```python
from build123d import *

# Parameters (mm, degrees)
SKETCH_1_R        = 1
EXTRUDE_1_DEPTH   = 3
SKETCH_2_R        = 4.35
SKETCH_2_R_2      = 3.35
EXTRUDE_1_2_DEPTH = 3


with BuildPart() as part:
    # 草图1 → Extrude 1 (new body)
    with BuildSketch(Plane.XY):
        with BuildLine():
            Line((-2.470698832, 13.581637634), (-3.604292918, 6.242818459))
            Line((-3.604292918, 6.242818459), (-10.5266938, 8.93050677))
            ThreePointArc((-10.5266938, 8.93050677), (-13.596598839, 7.85), (-12.997392632, 4.651130864))
            Line((-12.997392632, 4.651130864), (-7.208585836, 0))
            Line((-7.208585836, 0), (-12.997392632, -4.651130864))
            ThreePointArc((-12.997392632, -4.651130864), (-13.596598839, -7.85), (-10.5266938, -8.93050677))
            Line((-10.5266938, -8.93050677), (-3.604292918, -6.242818459))
            Line((-3.604292918, -6.242818459), (-2.470698832, -13.581637634))
            ThreePointArc((-2.470698832, -13.581637634), (0, -15.7), (2.470698832, -13.581637634))
            Line((2.470698832, -13.581637634), (3.604292918, -6.242818459))
            Line((3.604292918, -6.242818459), (10.5266938, -8.93050677))
            ThreePointArc((10.5266938, -8.93050677), (13.596598839, -7.85), (12.997392632, -4.651130864))
            Line((12.997392632, -4.651130864), (7.208585836, 0))
            Line((7.208585836, 0), (12.997392632, 4.651130864))
            ThreePointArc((12.997392632, 4.651130864), (13.596598839, 7.85), (10.5266938, 8.93050677))
            Line((10.5266938, 8.93050677), (3.604292918, 6.242818459))
            Line((3.604292918, 6.242818459), (2.470698832, 13.581637634))
            ThreePointArc((2.470698832, 13.581637634), (0, 15.7), (-2.470698832, 13.581637634))
        make_face()
        with Locations((6.495190528, 3.75)):
            Circle(SKETCH_1_R, mode=Mode.SUBTRACT)
        with Locations((0, 7.5)):
            Circle(SKETCH_1_R, mode=Mode.SUBTRACT)
        with Locations((6.495190528, -3.75)):
            Circle(SKETCH_1_R, mode=Mode.SUBTRACT)
        with Locations((0, -7.5)):
            Circle(SKETCH_1_R, mode=Mode.SUBTRACT)
        with Locations((-6.495190528, -3.75)):
            Circle(SKETCH_1_R, mode=Mode.SUBTRACT)
        with Locations((-6.495190528, 3.75)):
            Circle(SKETCH_1_R, mode=Mode.SUBTRACT)
    extrude(amount=EXTRUDE_1_DEPTH)

    # 草图2 → Extrude 1 2 (add)
    with BuildSketch(Plane.XY.offset(3)):
        Circle(SKETCH_2_R)
        Circle(SKETCH_2_R_2, mode=Mode.SUBTRACT)
    extrude(amount=EXTRUDE_1_2_DEPTH)


solid = part.part
```
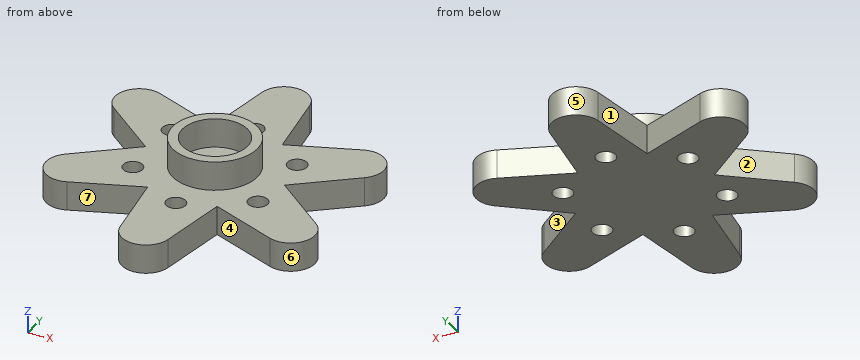
Geometry check sheet. Reference: the model listing, model coordinates, mm. Face numbers are marked on the shaded views. A direction names the side the tool comes from. Coordinates: 2 decimals unless noted, no trailing zeros. Order: outer loops, then holes, each group sorted by start corner. A loop starts at its lowest first (then second) coordinate and runs counter-clockwise, first axis right, second up. Notation, with made-up numbers: (1.5, -13) - (25.5, -13) arc R28 ccw to (25.5, 12) - close; hole circle Ø10 at (-8, 47.5). An arc over 180 degrees is marked (long way). Answer in a Markdown table with one row per item. Add a question column.
1. Section check A-A (z = 0.7). Enter the section's corners in (x, y), plus the area to 3 significant figures.
2. Gauge pin test, flat ends, axial feed: pin 1 Ø6 at (x, y) = (7.5, -5) entering from +Z; pin 2 Ø1.6 at (x, y) = (0, 7.5) entering from -Z. Record the tip position at first contact, or that the pin passes through.
3. Section check B-B (x = 0). Enter the section's corners in (y, z).
4. Draft check along Y on the marked faces 5, 6 and 7. Enter one of: +Y half, -Y half, draft (parallel to the pull), parting line (faces both ways), or undercut.
5. Section check D-D (y = -3.75). Enter the section's corners in (x, z), plus the area to 3 significant figures.
6. Section check C-C (x = -12). Enter the section's corners in (y, z).
7. Access from +Z, -Z, +X, -X, +Y, -Y to the whole of each face (thin tool, end or side, straight path). Record for the marked faces 1, 2, 3 and 4.
8. Material ranges on L1, parallel to Y at x = 0, z = 1.7; L2, parallel to X at y = -3.5, z = 1.8; L3, parallel to Y at x = -10, z = 0.8, recorded low to high. Write a range as [from, to].
Data:
| question | item | result |
|---|---|---|
| 1 | outline | (-13, -4.65) arc R2.5 ccw to (-10.53, -8.93) - (-3.6, -6.24) - (-2.47, -13.58) arc R2.5 ccw to (2.47, -13.58) - (3.6, -6.24) - (10.53, -8.93) arc R2.5 ccw to (13, -4.65) - (7.21, 0) - (13, 4.65) arc R2.5 ccw to (10.53, 8.93) - (3.6, 6.24) - (2.47, 13.58) arc R2.5 ccw to (-2.47, 13.58) - (-3.6, 6.24) - (-10.53, 8.93) arc R2.5 ccw to (-13, 4.65) - (-7.21, 0) - close; hole circle Ø2 at (-6.5, -3.75); hole circle Ø2 at (-6.5, 3.75); hole circle Ø2 at (0, -7.5); hole circle Ø2 at (0, 7.5); hole circle Ø2 at (6.5, -3.75); hole circle Ø2 at (6.5, 3.75) |
| 1 | area | 431 mm² |
| 2 | pin 1 | stops at z = 3 |
| 2 | pin 2 | passes through |
| 3 | outline | (-15.7, 0) - (-8.5, 0) - (-8.5, 3) - (-15.7, 3) - close; (-6.5, 0) - (6.5, 0) - (6.5, 3) - (4.35, 3) - (4.35, 6) - (3.35, 6) - (3.35, 3) - (-3.35, 3) - (-3.35, 6) - (-4.35, 6) - (-4.35, 3) - (-6.5, 3) - close; (8.5, 0) - (15.7, 0) - (15.7, 3) - (8.5, 3) - close |
| 4 | face 5 | +Y half |
| 4 | face 6 | undercut |
| 4 | face 7 | -Y half |
| 5 | outline | (-11.88, 0) - (-7.5, 0) - (-7.5, 3) - (-11.88, 3) - close; (-5.5, 0) - (5.5, 0) - (5.5, 3) - (2.2, 3) - (2.2, 6) - (-2.2, 6) - (-2.2, 3) - (-5.5, 3) - close; (7.5, 0) - (11.88, 0) - (11.88, 3) - (7.5, 3) - close |
| 5 | area | 72.5 mm² |
| 6 | outline | (-9.03, 0) - (-3.85, 0) - (-3.85, 3) - (-9.03, 3) - close; (3.85, 0) - (9.03, 0) - (9.03, 3) - (3.85, 3) - close |
| 7 | face 1 | +Z, -Z, +Y |
| 7 | face 2 | +Z, -Z, -X |
| 7 | face 3 | +Z, -Z, +X |
| 7 | face 4 | +Z, -Z, -Y |
| 8 | L1 | y = [-15.7, -8.5], [-6.5, 6.5], [8.5, 15.7] |
| 8 | L2 | x = [-11.56, -7.46], [-5.53, 5.53], [7.46, 11.56] |
| 8 | L3 | y = [-8.73, -2.24], [2.24, 8.73] |
